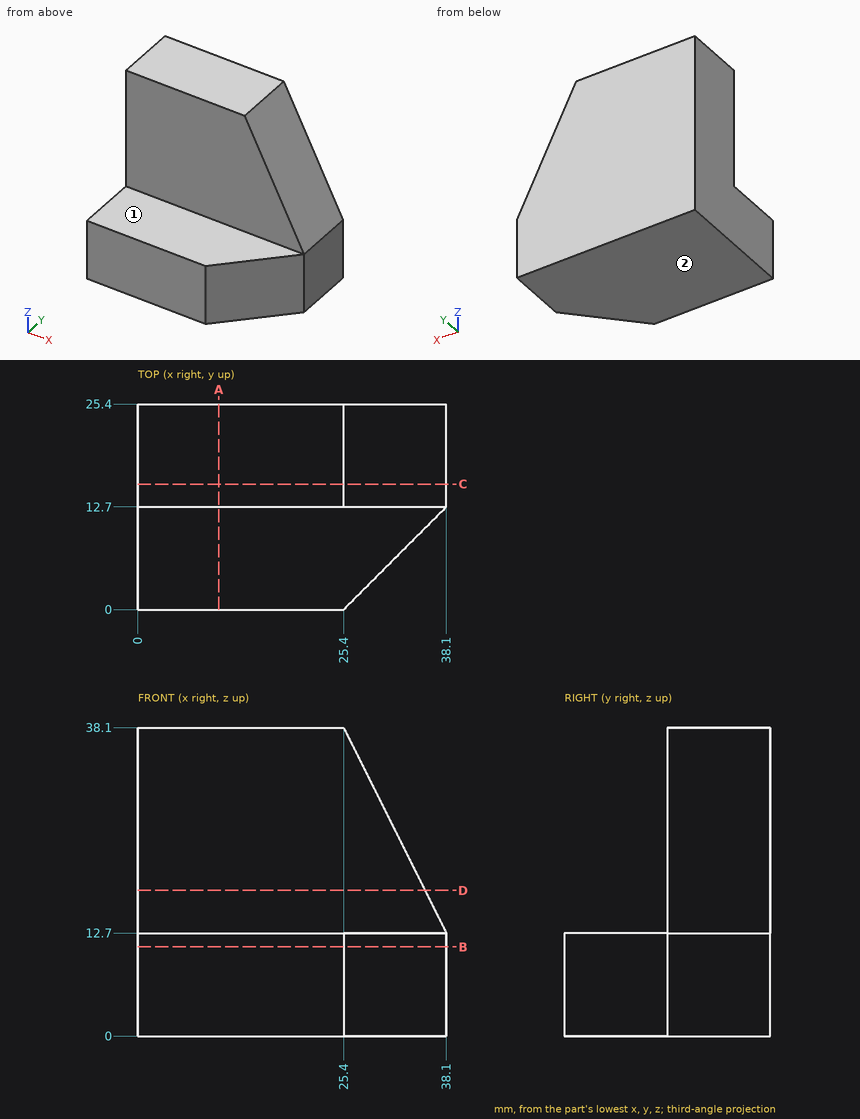
Could you check a few things on this drawing? It's one solid part, dimensions in mm from its lowest x, y, z. A direction names the side the tool comes from. Round coordinates to 2 decimals unless told otherwise and drop trailing zeros. Order: outer loops, then holes, each group sorted by start corner. A loop starts at its lowest first (then second) coordinate and runs counter-clockwise, first axis right, second up.
(1) Which directions (+Z, -Z, +X, -X, +Y, -Y) give clear straight access to the entire face, cutting with the end or side of a thin tool? Please do the marked faces 1 and 2.
Response values:
face 1: +Z, +X, -X, -Y
face 2: -Z, +X, -X, +Y, -Y
(2) Imagine slicing it at D-D (z = 18). Write out the boundary of the cut face in (x, y).
Response values:
outline: (0, 12.7) - (35.45, 12.7) - (35.45, 25.4) - (0, 25.4) - close
(3) Imagine slicing it at B-B (z = 11). Write out the boundary of the cut face in (x, y).
Response values:
outline: (0, 0) - (25.4, 0) - (38.1, 12.7) - (38.1, 25.4) - (0, 25.4) - close
(4) I'm going to push flat-ended pins straight in: pin 1 (8 mm diameter, centred on y = 16.5, z = 22, fed in from +X); pin 2 (10 mm diameter, centred on x = 11, y = 3, fed in from +Z); pin 3 (12.5 mm diameter, centred on x = 28, z = 25.5, fed in from -Y). Where does each tip first touch, or does it pass through?
Response values:
pin 1: stops at x = 35.45
pin 2: stops at z = 12.7
pin 3: stops at y = 12.7
(5) Imagine slicing it at A-A (x = 10). Write out the boundary of the cut face in (y, z), plus the area to 3 significant figures.
Response values:
outline: (0, 0) - (25.4, 0) - (25.4, 38.1) - (12.7, 38.1) - (12.7, 12.7) - (0, 12.7) - close
area: 645 mm2
(6) Please list where these lines run through material, in increasing order: line 1 along Y through (x, z) = (15, 35); line 2 along Z through (x, y) = (9, 7.25); line 3 along X through (y, z) = (6.5, 8).
Response values:
line 1: y = 12.7 to 25.4
line 2: z = 0 to 12.7
line 3: x = 0 to 31.9
(7) Imagine slicing it at C-C (y = 15.5). Write out the boundary of the cut face in (x, z), plus the area to 3 significant figures.
Response values:
outline: (0, 0) - (38.1, 0) - (38.1, 12.7) - (25.4, 38.1) - (0, 38.1) - close
area: 1,290 mm2
